Model file for the job. Use its own axes, mm. Face numbers are marked on the shaded views. A direction names the side the tool comes from. Round coordinates to 2 decimals unless told otherwise and drop trailing zeros. Order: outer loops, then holes, each group sorted by start corner. A loop starts at its lowest first (then second) coordinate and runs counter-clockwise, first axis right, second up. Notation, with made-up numbers: (-4, -8) - (7, -8) arc R15 cw to (7, 16) - close; hole circle Ø11 at (57, -19.75). An arc over 180 degrees is marked (long way). Write item = value, one per line.
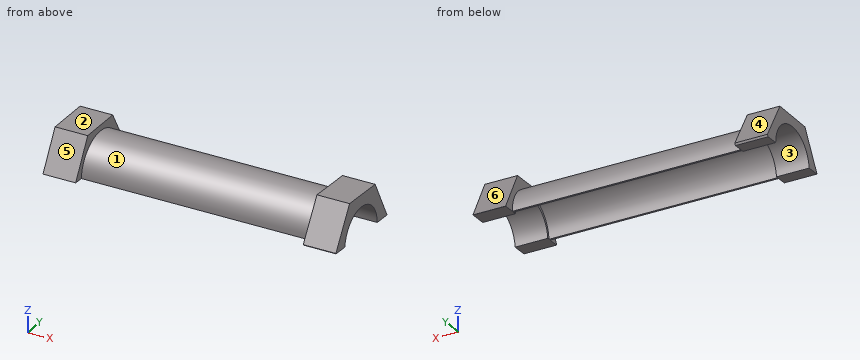
```python
from build123d import *

# Parameters (mm, degrees)
SKETCH1_R            = 50.800375113
SKETCH1_R_2          = 47.812951641
BOSS_EXTRUDE2_DEPTH  = 350
BOSS_EXTRUDE5_DEPTH  = 50
BOSS_EXTRUDE11_DEPTH = 50
SKETCH6_R            = 44.996318031
CUT_EXTRUDE2_DEPTH   = 50
SKETCH7_R            = 43.517898498
CUT_EXTRUDE3_DEPTH   = 50
CUT_EXTRUDE5_DEPTH   = 460.276368741


with BuildPart() as part:
    # Sketch1 → Boss-Extrude2 (new body)
    with BuildSketch(Plane(origin=(0, 0, 0), x_dir=(0, 0, -1), z_dir=(1, 0, 0))):
        with Locations((1.289702318, 0)):
            Circle(SKETCH1_R)
        with Locations((1.289702318, 0)):
            Circle(SKETCH1_R_2, mode=Mode.SUBTRACT)
    extrude(amount=BOSS_EXTRUDE2_DEPTH)

    # Sketch3 → Boss-Extrude5 (add)
    with BuildSketch(Plane(origin=(350, 0, 0), x_dir=(0, 0, -1), z_dir=(1, 0, 0))):
        Polygon((58.055626726, -36.855405481), (60.945530776, 31.849944836), (2.88990405, 68.705350317), (-58.055626726, 36.855405481), (-60.945530776, -31.849944836), (-2.88990405, -68.705350317), align=None)
        Polygon((29.411876605, -18.99044871), (30.315925302, 11.383738416), (4.46313198, 27.353761118), (-22.293710039, 12.949596693), (-23.197758737, -17.424590433), (2.655034585, -33.394613135), align=None, mode=Mode.SUBTRACT)
    extrude(amount=BOSS_EXTRUDE5_DEPTH)

    # Sketch5 → Boss-Extrude11 (add)
    with BuildSketch(Plane.ZY):
        Polygon((0, -67.161353017), (58.163437865, -33.580676508), (58.163437865, 33.580676508), (0, 67.161353017), (-58.163437865, 33.580676508), (-58.163437865, -33.580676508), align=None)
    extrude(amount=BOSS_EXTRUDE11_DEPTH)

    # Sketch6 → Cut-Extrude2 (cut)
    with BuildSketch(Plane(origin=(0, 0, 0), x_dir=(0, 0, -1), z_dir=(1, 0, 0))):
        with Locations((2.167278034, 0)):
            Circle(SKETCH6_R)
    extrude(amount=-CUT_EXTRUDE2_DEPTH, mode=Mode.SUBTRACT)

    # Sketch7 → Cut-Extrude3 (cut)
    with BuildSketch(Plane.ZY.offset(-350)):
        with Locations((-2.231478452, -1.09442532)):
            Circle(SKETCH7_R)
    extrude(amount=-CUT_EXTRUDE3_DEPTH, mode=Mode.SUBTRACT)

    # Sketch9 → Cut-Extrude5 (cut, through all)
    with BuildSketch(Plane(origin=(400, 0, 0), x_dir=(0, 0, -1), z_dir=(1, 0, 0))):
        Polygon((3.435375401, 77.5085151), (88.372603531, 77.5085151), (88.372603531, -82.273926917), (-2.672776716, -84.939108123), align=None)
    extrude(amount=-CUT_EXTRUDE5_DEPTH, mode=Mode.SUBTRACT)


solid = part.part
```
1) Cut at D-D (y = 10.5). Write the cut outline in (x, z).
Conclusion:
outline = (-50, 41.59) - (0, 41.59) - (0, 45.36) - (350, 45.36) - (350, 39.71) - (400, 39.71) - (400, 59.16) - (350, 59.16) - (350, 48.41) - (0, 48.41) - (0, 58.16) - (-50, 58.16) - close
2) Flat gauge pins, fed straight in: pin 1 Ø10 at (x, z) = (349, 16.5) entering from -Y; pin 2 Ø15 at (x, y) = (-35.5, -15.5) entering from +Z; pin 3 Ø3 at (x, z) = (214, 47) entering from -Y. Where does each tip first touch, or does it go through?
Conclusion:
pin_1 = -63.18
pin_2 = 58.16
pin_3 = -19.78
3) Cut at A-A (z = 33.5). Write the cut outline in (x, y).
Conclusion:
outline = (-50, -47.82) - (0, -47.82) - (0, -37.02) - (350, -37.02) - (350, -49.27) - (400, -49.27) - (400, -25.94) - (350, -25.94) - (350, -32.8) - (0, -32.8) - (0, -27.43) - (-50, -27.43) - close; (-50, 27.43) - (0, 27.43) - (0, 32.8) - (350, 32.8) - (350, 23.75) - (400, 23.75) - (400, 49.69) - (350, 49.69) - (350, 37.02) - (0, 37.02) - (0, 47.82) - (-50, 47.82) - close
4) 3-axis set-ups, long thin cutter, end or side, ignore diameter. For the marked faces 4, 5 and 6: which of +Z, -Z, +X, -X, +Y, -Y reach the whole face in a straight line?
Conclusion:
face_4 = +Z, -X, +Y
face_5 = +Z, -X, -Y
face_6 = +Z, +X, -X, +Y
5) Mould opens along Y. For the marked faces 1, 2 and 3 say: +Y half, -Y half, draft (parallel to the pull), parting line (faces both ways), or undercut.
Conclusion:
face_1 = parting line
face_2 = draft
face_3 = undercut
6) Wall check: line 1 along X through (y, z) = (32, 47); line 2 along Y through (x, z) = (329.5, 1.5); line 3 along Y through (x, z) = (219, 20). Give the ranges that are in metal, low to high.
Conclusion:
line_1 = -50 to 0, 350 to 400
line_2 = -50.72 to -47.73, 47.73 to 50.72
line_3 = -46.12 to -42.81, 42.81 to 46.12
7) Cut at B-B (y = -11). Write the cut outline in (x, z).
Conclusion:
outline = (-50, 41.46) - (0, 41.46) - (0, 45.24) - (350, 45.24) - (350, 40.14) - (400, 40.14) - (400, 60.07) - (350, 60.07) - (350, 48.31) - (0, 48.31) - (0, 58.16) - (-50, 58.16) - close
8) Cut at C-C (x = -11). Write the cut outline in (y, z).
Conclusion:
outline = (-66.03, 1.96) - (-44.87, 1.17) arc R45 cw to (45, -2.21) - (65.44, -2.98) - (67.16, 0) - (33.58, 58.16) - (-33.58, 58.16) - close
